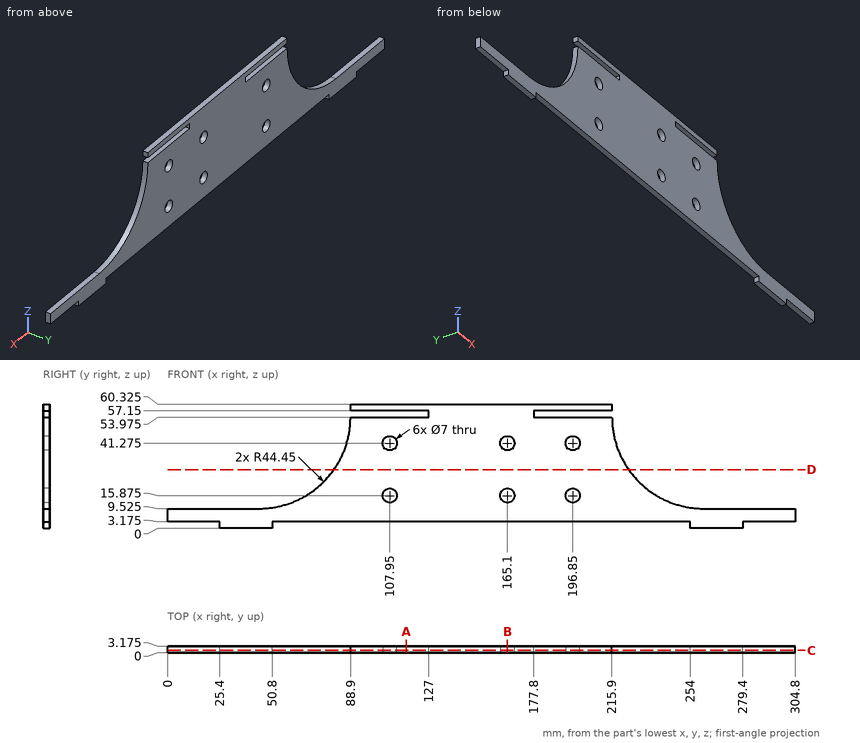
Can you work these out from the drawing? Everything is in mm from the part's minimum corner. Round coordinates to 2 decimals unless told otherwise and drop trailing zeros. Write each loop counter-clockwise with the first axis right and the second up, starting at its lowest first coordinate (ties: lowest second). Pieces come first, ordered by that corner, then holes. Notation, with made-up numbers: M 42.25,45.25 L 57.25,45.25 A31 ccw 57.25,73.25 Z; hole C 60.25,30 d1. An arc over 180 degrees is marked long. Use a Markdown table: item, result.
Item 1: I want a section at C-C (y = 1.1). State how many separate pieces and enclosed holes the cut face has, and give its area (3 significant figures).
Found:
| item | result |
|---|---|
| separate pieces | 1 |
| enclosed holes | 6 |
| area | 8,920 mm2 |
Item 2: If I drill on line 1 along Z through (x, y) = (196.85, 1.5) (3 decimals); line 2 along Z through (x, y) = (165.1, 2.3) (3 decimals); line 3 along Z through (x, y) = (187, 1.15) (3 decimals), over which ranges is the centre line in solid material (lowest first)? Write a range as [from, to].
Found:
| item | result |
|---|---|
| line 1 | z = [3.175, 12.375], [19.375, 37.775], [44.775, 53.975], [57.15, 60.325] |
| line 2 | z = [3.175, 12.375], [19.375, 37.775], [44.775, 60.325] |
| line 3 | z = [3.175, 53.975], [57.15, 60.325] |
Item 3: For pin 1 Ø1 at (y, z) = (2.5, 55.5) entering from -X; pin 2 Ø1 at (x, y) = (18.5, 1.5) entering from -Z (3 decimals); pin 3 Ø1 at (y, z) = (2, 1) entering from +X, each with a flat end and sliding along its axis, tell me the tip position at first contact or that it passes through.
Found:
| item | result |
|---|---|
| pin 1 | stops at x = 127 |
| pin 2 | stops at z = 3.175 |
| pin 3 | stops at x = 279.4 |
Item 4: I want a section at D-D (z = 28.5). List the corners of the cut face in (x, y) for me (3 decimals).
Found:
| item | result |
|---|---|
| outline | M 80.876,0 L 223.924,0 L 223.924,3.175 L 80.876,3.175 Z |
Item 5: I want a section at B-B (x = 165.1). List the corners of the cut face in (y, z) for me (3 decimals).
Found:
| item | result |
|---|---|
| outline | M 0,3.175 L 3.175,3.175 L 3.175,12.375 L 0,12.375 Z; M 0,19.375 L 3.175,19.375 L 3.175,37.775 L 0,37.775 Z; M 0,44.775 L 3.175,44.775 L 3.175,60.325 L 0,60.325 Z |
Item 6: I want a section at A-A (x = 116). List the corners of the cut face in (y, z) for me (3 decimals).
Found:
| item | result |
|---|---|
| outline | M 0,3.175 L 3.175,3.175 L 3.175,53.975 L 0,53.975 Z; M 0,57.15 L 3.175,57.15 L 3.175,60.325 L 0,60.325 Z |
